Source: three-view drawing plus pictorial views. Frame: mm from the lowest corner of the part. Round coordinates to 2 decimals unless told otherwise and drop trailing zeros. Order: outer loops, then holes, each group sorted by start corner. A loop starts at its lowest first (then second) coordinate and runs counter-clockwise, first axis right, second up. Notation, with made-up numbers: (76.25, 83) -> (108.25, 83) arc R18 ccw to (108.25, 113) -> close; hole circle Ø4 at (-4.75, 49.25). An arc over 180 degrees is marked (long way). Answer as CSV lines item,"result". Start each with the question number.
1) Line query: L1, parallel to Y at x = 50.5, z = 4.4; L2, parallel to Y at x = 12.5, z = 2.9 (1 decimal); L3, parallel to Z at x = 50, y = 7.75. Output: solid intervals per line, ascending.
2) Mould query, pull axis Y, two halves, no side actions, for the marked faces 1, 2 and 3. Classes: +Y half, -Y half, draft (parallel to the pull), parting line (faces both ways), or undercut.
3) Section query B-B, the plane y = 1. Output: boundary loops of the cut face in (x, z).
4) Section query C-C, the plane z = 2.5. Output: boundary loops of the cut face in (x, y), and give its area (3 significant figures).
5) Section query A-A, the plane x = 4.5. Output: boundary loops of the cut face in (y, z).
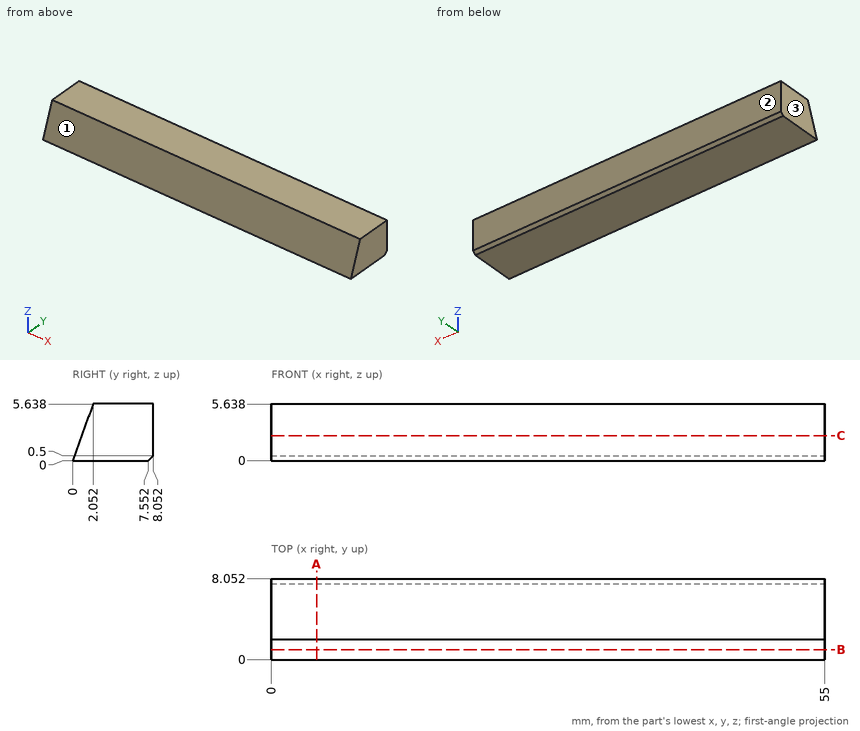
Findings:
1,L1,"y = 1.6 to 8.05"
1,L2,"y = 1.1 to 8.1"
1,L3,"z = 0.2 to 5.64"
2,face 1,"-Y half"
2,face 2,"+Y half"
2,face 3,"draft"
3,outline,"(0, 0) -> (55, 0) -> (55, 2.75) -> (0, 2.75) -> close"
4,outline,"(0, 0.91) -> (55, 0.91) -> (55, 8.05) -> (0, 8.05) -> close"
4,area,"393 mm^2"
5,outline,"(0, 0) -> (7.55, 0) -> (8.05, 0.5) -> (8.05, 5.64) -> (2.05, 5.64) -> close"
